```python
from build123d import *

# Parameters (mm, degrees)
BASE_FLANGE1_DEPTH       = 1.5875
EDGE_FLANGE1_START       = -2.38125
EDGE_FLANGE1_OUTLINE_W   = 0.79375
EDGE_FLANGE1_OUTLINE_H   = 1.5875
EDGE_FLANGE1_DEPTH       = 2.38125
EDGE_FLANGE1_START_2     = 74.6125
EDGE_FLANGE1_2_OUTLINE_W = 190.5
EDGE_FLANGE1_2_OUTLINE_H = 50.8
EDGE_FLANGE1_2_DEPTH     = 3.175
EDGE_FLANGE1_START_3     = 76.2
EDGE_FLANGE1_3_OUTLINE_W = 190.5
EDGE_FLANGE1_3_OUTLINE_H = 1.5875
EDGE_FLANGE1_3_DEPTH     = 1.2613005
EDGE_FLANGE1_START_4     = 152.4
EDGE_FLANGE1_4_DEPTH     = 190.5


with BuildPart() as part:
    # Base-Flange1: sheet metal written as solids
    # Sketch1 → Base-Flange1 (new body)
    with BuildSketch(Plane(origin=(0, 0, 0), x_dir=(1, 0, 0), z_dir=(0, 1, 0))):
        Polygon((0, 0), (495.3, 0), (495.3, -50.8), (419.1, -50.8), (419.1, -177.8), (342.9, -177.8), (342.9, -76.2), (152.4, -76.2), (152.4, -177.8), (76.2, -177.8), (76.2, -50.8), (0, -50.8), align=None)
    extrude(amount=-BASE_FLANGE1_DEPTH)

    # Edge-Flange1: read off the stored shape, not the designer's step
    # Edge-Flange1 outline → Edge-Flange1 (cut)
    with BuildSketch(Plane(origin=(0, -1.5875, 76.2), x_dir=(-1, 0, 0), z_dir=(0, 0, 1)).offset(EDGE_FLANGE1_START)):
        with Locations((-152.003125, -0.79375)):
            Rectangle(EDGE_FLANGE1_OUTLINE_W, EDGE_FLANGE1_OUTLINE_H)
        with Locations((-343.296875, -0.79375)):
            Rectangle(EDGE_FLANGE1_OUTLINE_W, EDGE_FLANGE1_OUTLINE_H)
    extrude(amount=EDGE_FLANGE1_DEPTH, mode=Mode.SUBTRACT)

    # Edge-Flange1 2 outline → Edge-Flange1 2 (add)
    with BuildSketch(Plane.XY.offset(EDGE_FLANGE1_START_2)):
        with Locations((247.65, -26.9875)):
            Rectangle(EDGE_FLANGE1_2_OUTLINE_W, EDGE_FLANGE1_2_OUTLINE_H)
    extrude(amount=EDGE_FLANGE1_2_DEPTH)

    # Edge-Flange1 3 outline → Edge-Flange1 3 (add)
    with BuildSketch(Plane.XY.offset(EDGE_FLANGE1_START_3)):
        with Locations((247.65, -0.79375)):
            Rectangle(EDGE_FLANGE1_3_OUTLINE_W, EDGE_FLANGE1_3_OUTLINE_H)
    extrude(amount=EDGE_FLANGE1_3_DEPTH)

    # Edge-Flange1 4 outline → Edge-Flange1 4 (cut)
    with BuildSketch(Plane.YZ.offset(EDGE_FLANGE1_START_4)):
        with BuildLine():
            Line((-3.175, 76.2), (-52.3875, 76.2))
            Line((-52.3875, 76.2), (-52.3875, 74.6125))
            Line((-52.3875, 74.6125), (-1.5875, 74.6125))
            ThreePointArc((-1.5875, 74.6125), (-2.052467985, 75.735032015), (-3.175, 76.2))
        make_face()
        with BuildLine():
            Line((-1.5875, 77.7875), (-3.175, 77.7875))
            ThreePointArc((-3.175, 77.7875), (-0.92993597, 76.85756403), (0, 74.6125))
            Line((0, 74.6125), (0, 77.4613005))
            Line((0, 77.4613005), (-1.5875, 77.4613005))
            Line((-1.5875, 77.4613005), (-1.5875, 77.7875))
        make_face()
    extrude(amount=EDGE_FLANGE1_4_DEPTH, mode=Mode.SUBTRACT)


solid = part.part
```
Geometry check sheet. Reference: the model listing, model coordinates, mm. A direction names the side the tool comes from. Give positions to 0.01 mm unless a question says otherwise; leave off trailing zeros. Loops run counter-clockwise (first coordinate to the right, second up) from the corner with the lowest first, then second, coordinate; pieces in that order, holes last. Notation, with made-up numbers: M 6,-33 L 60,-33 A20 cw 60,-10 Z; hole C 15,-15 d5. An arc over 180 degrees is marked long. Answer as CSV lines item,"result".
Item 1: Access from +Z, -Z, +X, -X, +Y, -Y to the whole of each face (thin tool, end or side, straight path). Record for faces 1 (the flat face through (244, 0, 68)), 2 (the flat face through (246, -27, 76.2)).
Values:
face 1,"+Z, -Z, +X, -X, +Y"
face 2,"-Z, +X, -X, -Y"
Item 2: Cross-section at C-C on y = -26. Record the cut outline in (x, z).
Values:
outline,"M 152.4,76.2 L 342.9,76.2 L 342.9,77.79 L 152.4,77.79 Z"
Item 3: Cross-section at D-D on z = 28.5. Record the cut outline in (x, y), and give its area (3 significant figures).
Values:
outline,"M 0,-1.59 L 495.3,-1.59 L 495.3,0 L 0,0 Z"
area,"786 mm²"
Item 4: Depth check by flat-ended pin: P1, Ø1, axis at x = 333, y = -7.5, coming from the -Z side; P2, Ø1.3, axis at y = -1, z = 137.5, coming from the -X side; P3, Ø8, axis at y = -9, z = 74, coming from the +X side; P4, Ø12, axis at x = 390, y = -12, coming from the -Z side. Enter the tip coordinate at first touch or a pass-through.
Values:
P1,"stops at z = 76.2"
P2,"stops at x = 76.2"
P3,"stops at x = 342.9"
P4,"passes through"
Item 5: Cross-section at A-A on z = 153.5. Record the cut outline in (x, y).
Values:
outline,"M 76.2,-1.59 L 152.4,-1.59 L 152.4,0 L 76.2,0 Z; M 342.9,-1.59 L 419.1,-1.59 L 419.1,0 L 342.9,0 Z"
Item 6: Material ranges on line 1 (Y direction, x = 131.5, z = 103); line 2 (Z direction, x = 186, y = -39.5), recorded low to high.
Values:
line 1,"y = -1.59 to 0"
line 2,"z = 76.2 to 77.79"
